from build123d import *

# Parameters (mm, degrees)
EXTRUDE_1_DEPTH            = 10
HOLE_WIZARD_M41_D          = 4.5
HOLE_WIZARD_M41_DEPTH      = 9.8
M4X0_71_D                  = 3.3
HOLE_WIZARD_1_4_201_REACH  = 48.271
HOLE_WIZARD_1_4_201_BORE_R = 2.5527
FILLET_1_R                 = 2


with BuildPart() as part:
    # Эскиз1 → Бобышка-Вытянуть1 (new body)
    with BuildSketch(Plane.XY):
        with BuildLine():
            Line((10.220689801, 4.2), (21, 4.2))
            Line((21, 4.2), (21, 14))
            Line((21, 14), (0, 14))
            ThreePointArc((0, 14), (-9.899494937, 9.899494937), (-14, 0))
            Line((-14, 0), (-14, -26))
            Line((-14, -26), (7, -26))
            ThreePointArc((7, -26), (16.899494937, -21.899494937), (21, -12))
            Line((21, -12), (21, 0))
            Line((21, 0), (11.05, 0))
            ThreePointArc((11.05, 0), (-10.840690068, -2.140546391), (10.220689801, 4.2))
        make_face()
    extrude(amount=EXTRUDE_1_DEPTH)

    # Отверстие с зазором M41
    with Locations(Plane(origin=(0, 14, 0), x_dir=(1, 0, 0), z_dir=(0, 1, 0))):
        with Locations((16, -5)):
            Hole(HOLE_WIZARD_M41_D / 2, depth=HOLE_WIZARD_M41_DEPTH)

    # Отверстие обработанное метчиком M4x0.71 (through all)
    with Locations(Plane(origin=(0, 0, 0), x_dir=(1, 0, 0), z_dir=(0, 1, 0))):
        with Locations((16, -5)):
            Hole(M4X0_71_D / 2)

    # Отверстие обработанное метчиком 1/4-201 bore → Отверстие обработанное метчиком 1/4-201 (cut, up to next)
    with BuildSketch(Plane(origin=(0, -26, 0), x_dir=(-1, 0, 0), z_dir=(0, -1, 0)), mode=Mode.PRIVATE) as hole_wizard_1_4_201_sk1:
        with Locations((7, -5)):
            Circle(HOLE_WIZARD_1_4_201_BORE_R)
    hole_wizard_1_4_201_tool1 = extrude(hole_wizard_1_4_201_sk1.sketch, amount=-HOLE_WIZARD_1_4_201_REACH, mode=Mode.PRIVATE) & part.part
    add(hole_wizard_1_4_201_tool1.solids().sort_by_distance((-7, -26, 5))[0], mode=Mode.SUBTRACT)

    # Скругление1
    fillet_1_edges = [part.edges().sort_by_distance(p)[0] for p in [
        (11.05, 0, 5),
        (21, 0, 5),
        (-14, -26, 5),
        (21, 14, 5),
        (21, 4.2, 5),
        (10.220689801, 4.2, 5),
    ]]
    fillet(fillet_1_edges, radius=FILLET_1_R)


solid = part.part
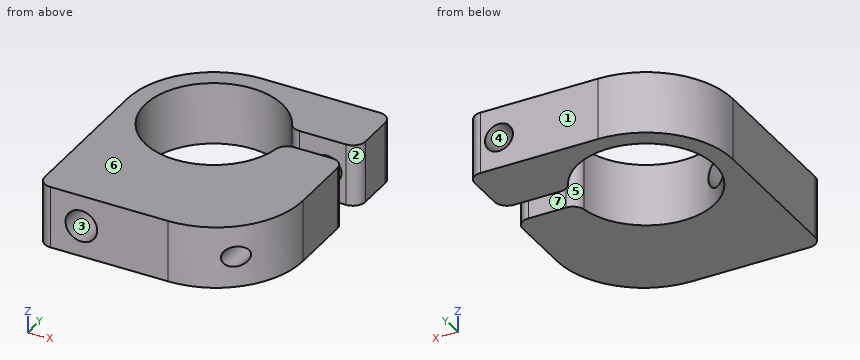
Could you check a few things on this model? Use its own coordinates, in mm. Face numbers are marked on the shaded views. A direction names the side the tool comes from. Give positions to 0.01 mm unless a question says otherwise; leave off trailing zeros. Order: outer loops, then holes, each group sorted by start corner. A loop starts at its lowest first (then second) coordinate and runs counter-clockwise, first axis right, second up. Notation, with made-up numbers: (-16.5, 10) - (6.5, 10) arc R10 cw to (6.5, 17) - close; hole circle Ø10 at (83.5, 39). An arc over 180 degrees is marked (long way). Return JSON: item names as keys, results as strings. Group by question number.
Q1. Suppose I cut it at B-B, the plane z = 9. Please give me the cut outline in (x, y).
Q2. Which directions (+Z, -Z, +X, -X, +Y, -Y) give clear straight access to the entire face, cutting with the end or side of a thin tool? Please do the marked faces 4, 5, 6 and 7.
Q3. Suppose I cut it at D-D, the plane x = 16. Please give me the cut outline in (y, z).
Q4. Will these pins go through, and if not, where does the flat tip stop? pin 1 Ø4 at (x, z) = (14, 6) entering from -Y; pin 2 Ø1.5 at (x, z) = (16.5, 6) entering from +Y; pin 3 Ø3 at (x, z) = (-4.5, 6.5) entering from +Y; pin 4 Ø10 at (x, y) = (9, -6.5) entering from -Z.
Q5. Suppose I cut it at A-A, the plane y = -8. Please give me the cut outline in (x, z), and give its area (3 significant figures).
Q6. Please list where these lines run through material, in increasing order: line 1 along Z through (x, y) = (16, 7); line 2 along Z through (x, y) = (16, -10.75); line 3 along X through (y, z) = (-9, 5). Write a range as [from, to].
Q7. Thinking about a two-plate mould opening in Y: for the marked faces 1, 2 and 3, which applies, pulls with the +Y half, pulls with the -Y half, needs draft (parallel to the pull), parting line crosses it, or undercut?
Q8. Suppose I cut it at C-C, the plane x = -5. Please give me the cut outline in (y, z).
Resolved:
{
 "1": {"outline": "(-14, -24) arc R2 ccw to (-12, -26) - (7, -26) arc R14 ccw to (21, -12) - (21, -2) arc R2 ccw to (19, 0) - (12.9, 0) arc R2 ccw to (10.92, -1.69) arc R11.05 cw (long way) to (9.72, 5.25) arc R2 ccw to (11.48, 4.2) - (19, 4.2) arc R2 ccw to (21, 6.2) - (21, 12) arc R2 ccw to (19, 14) - (0, 14) arc R14 ccw to (-14, 0) - close"},
 "2": {"face 4": "+Y", "face 5": "+Z, -Z", "face 6": "+Z, +X, -X, +Y, -Y", "face 7": "+Z, -Z, +X"},
 "3": {"outline": "(-22.72, 0) - (0, 0) - (0, 3.35) - (-22.72, 3.35) - close; (-22.72, 6.65) - (0, 6.65) - (0, 10) - (-22.72, 10) - close; (4.2, 0) - (14, 0) - (14, 2.75) - (4.2, 2.75) - close; (4.2, 7.25) - (14, 7.25) - (14, 10) - (4.2, 10) - close"},
 "4": {"pin 1": "stops at y = -25.08", "pin 2": "stops at y = 0", "pin 3": "stops at y = 13.67", "pin 4": "stops at z = 0"},
 "5": {"outline": "(-14, 0) - (-7.62, 0) - (-7.62, 2.52) arc R2.55 cw to (-7.62, 7.48) - (-7.62, 10) - (-14, 10) - close; (7.62, 0) - (21, 0) - (21, 10) - (7.62, 10) - close; hole circle Ø3.3 at (16, 5)", "area": "182 mm2"},
 "6": {"line 1": "z = [0, 2.75], [7.25, 10]", "line 2": "z = [0, 3.35], [6.65, 10]", "line 3": "x = [-14, -9.55], [6.41, 14.35], [17.65, 21]"},
 "7": {"face 1": "pulls with the +Y half", "face 2": "undercut", "face 3": "needs draft"},
 "8": {"outline": "(-26, 0) - (-9.85, 0) - (-9.85, 3.41) - (-26, 3.41) - close; (-26, 6.59) - (-9.85, 6.59) - (-9.85, 10) - (-26, 10) - close; (9.85, 0) - (13.08, 0) - (13.08, 10) - (9.85, 10) - close"}
}
